Build history of the part. All positions in model axes, mm. A direction names the side the tool comes from. Coordinates: 2 decimals unless noted, no trailing zeros. Order: outer loops, then holes, each group sorted by start corner. A loop starts at its lowest first (then second) coordinate and runs counter-clockwise, first axis right, second up. Notation, with made-up numbers: (4, -35.5) -> (47, -35.5) arc R20 ccw to (47, -15.5) -> close; hole circle Ø5 at (52, 32). An arc over 180 degrees is marked (long way). Write each question's results on one line, items separated by ' | '.
from build123d import *

# Parameters (mm, degrees)
BOSS_EXTRUDE1_DEPTH = 17.5
SKETCH4_OUTSIDE_W   = 245.87
SKETCH4_OUTSIDE_H   = 80.87
SKETCH4_OUTSIDE_W_2 = 115
SKETCH4_OUTSIDE_H_2 = 16
CUT_EXTRUDE1_DEPTH  = 48
SKETCH5_W           = 35
SKETCH5_H           = 35
BOSS_EXTRUDE2_DEPTH = 50
SKETCH6_R           = 4.25
CUT_EXTRUDE2_DEPTH  = 122.671689394


with BuildPart() as part:
    # Sketch1 → Boss-Extrude1 (new, symmetric)
    with BuildSketch(Plane.XY):
        Polygon((-100, 0), (100, 0), (100, 10), (65, 10), (65, 35), (57.5, 35), (57.5, 83), (-57.5, 83), (-57.5, 35), (-65, 35), (-65, 10), (-100, 10), align=None)
    extrude(amount=BOSS_EXTRUDE1_DEPTH, both=True)

    # Sketch4 outside → Cut-Extrude1 (cut)
    with BuildSketch(Plane(origin=(0, 83, 0), x_dir=(1, 0, 0), z_dir=(0, 1, 0))):
        Rectangle(SKETCH4_OUTSIDE_W, SKETCH4_OUTSIDE_H)
        Rectangle(SKETCH4_OUTSIDE_W_2, SKETCH4_OUTSIDE_H_2, mode=Mode.SUBTRACT)
    extrude(amount=-CUT_EXTRUDE1_DEPTH, mode=Mode.SUBTRACT)

    # Sketch5 → Boss-Extrude2 (add, symmetric)
    with BuildSketch(Plane.XY):
        with Locations((-12.5, 17.5)):
            Rectangle(SKETCH5_W, SKETCH5_H)
    extrude(amount=BOSS_EXTRUDE2_DEPTH, both=True)

    # Sketch6 → Cut-Extrude2 (cut, through all)
    with BuildSketch(Plane(origin=(0, 35, 0), x_dir=(1, 0, 0), z_dir=(0, 1, 0))):
        with Locations(Location((-12.5, -33.75, 0), (0, 0, 270))):
            Circle(SKETCH6_R)
        with Locations(Location((-82.75, 0, 0), (0, 0, 270))):
            Circle(SKETCH6_R)
        with Locations(Location((82.75, 0, 0), (0, 0, 270))):
            Circle(SKETCH6_R)
        with Locations(Location((-12.5, 33.75, 0), (0, 0, 90))):
            Circle(SKETCH6_R)
    extrude(amount=-CUT_EXTRUDE2_DEPTH, mode=Mode.SUBTRACT)


solid = part.part
Item 1: Tool access for faces 1 (the flat face through (-57.5, 59, 0)), 2 (the flat face through (-58, 14, -17.5)), 3 (the flat face through (-30, 17, 34)): list every direction of +Z, -Z, +X, -X, +Y, -Y with a clear straight run to the whole face (end or side of a thin tool).
Answer:
face 1: +Z, -Z, -X, +Y | face 2: -Z, -X, +Y, -Y | face 3: +Z, -X, +Y, -Y
Item 2: Pull direction Z, two halves, no side cores. Call faces 4 (the flat face through (65, 22, 0)), 5 (the flat face through (41, 18, -17.5)), 6 (the cylindrical face through (-86.5, 5.1, 2)): released by +Z, released by -Z, zero draft, split by the parting line, or undercut.
Answer:
face 4: zero draft | face 5: released by -Z | face 6: undercut
Item 3: Slice it at C-C, the plane z = -33.75. List the corners of the cut face in (x, y).
Answer:
outline: (-30, 0) -> (-16.75, 0) -> (-16.75, 35) -> (-30, 35) -> close; (-8.25, 0) -> (5, 0) -> (5, 35) -> (-8.25, 35) -> close
Item 4: Slice it at A-A, the plane x = -12.5. List the corners of the cut face in (y, z), and give its area (3 significant figures).
Answer:
outline: (0, -50) -> (35, -50) -> (35, -38) -> (0, -38) -> close; (0, -29.5) -> (35, -29.5) -> (35, -8) -> (83, -8) -> (83, 8) -> (35, 8) -> (35, 29.5) -> (0, 29.5) -> close; (0, 38) -> (35, 38) -> (35, 50) -> (0, 50) -> close | area: 3,670 mm^2
Item 5: Slice it at B-B, the plane z = 0. List the corners of the cut face in (x, y).
Answer:
outline: (-100, 0) -> (-87, 0) -> (-87, 10) -> (-100, 10) -> close; (-78.5, 0) -> (78.5, 0) -> (78.5, 10) -> (65, 10) -> (65, 35) -> (57.5, 35) -> (57.5, 83) -> (-57.5, 83) -> (-57.5, 35) -> (-65, 35) -> (-65, 10) -> (-78.5, 10) -> close; (87, 0) -> (100, 0) -> (100, 10) -> (87, 10) -> close
Item 6: Drill centre lines: line 1 (X direction, y = 2, z = 0); line 2 (X direction, y = 19, z = 33.75); line 3 (Z direction, x = 17, y = 54). Where is each one in solid material? Low to high. Write a range as from..to.
Answer:
line 1: x = -100..-87, -78.5..78.5, 87..100 | line 2: x = -30..-16.75, -8.25..5 | line 3: z = -8..8
Item 7: Slice it at D-D, the plane y = 18. List the corners of the cut face in (x, z), and give its area (3 significant figures).
Answer:
outline: (-65, -17.5) -> (-30, -17.5) -> (-30, -50) -> (5, -50) -> (5, -17.5) -> (65, -17.5) -> (65, 17.5) -> (5, 17.5) -> (5, 50) -> (-30, 50) -> (-30, 17.5) -> (-65, 17.5) -> close; hole circle Ø8.5 at (-12.5, -33.75); hole circle Ø8.5 at (-12.5, 33.75) | area: 6,710 mm^2
Item 8: Pin check, flat tips, straight feed: pin 1 (5 mm diameter, centred on x = -9.5, z = 39.5, fed in from +Y); pin 2 (4 mm diameter, centred on x = 38.5, y = 45, fed in from +Z); pin 3 (10.5 mm diameter, centred on x = -70.5, y = 13.5, fed in from +Z); pin 4 (1 mm diameter, centred on x = -46.5, z = -10, fed in from -Y). Stop position of each tip, or through.
Answer:
pin 1: stops at y = 35 | pin 2: stops at z = 8 | pin 3: stops at z = 17.5 | pin 4: stops at y = 0
